from build123d import *

# Parameters (mm, degrees)
SKETCH1_W           = 40
SKETCH1_H           = 30
SKETCH1_W_2         = 34
SKETCH1_H_2         = 24
EXTRUDE_THIN1_DEPTH = 330
EXTRUDE1_DEPTH      = 41
EXTRUDE2_DEPTH      = 33.318373456


with BuildPart() as part:
    # Sketch1 → Extrude-Thin1 (new body)
    with BuildSketch(Plane(origin=(0, 0, 0), x_dir=(1, 0, 0), z_dir=(0, 1, 0))):
        Rectangle(SKETCH1_W, SKETCH1_H)
        Rectangle(SKETCH1_W_2, SKETCH1_H_2, mode=Mode.SUBTRACT)
    extrude(amount=EXTRUDE_THIN1_DEPTH)

    # Sketch2 → Extrude1 (cut, through all)
    with BuildSketch(Plane.ZY.offset(20)):
        Polygon((-15, 330), (15, 330), (15, 318.182685732), align=None)
    extrude(amount=-EXTRUDE1_DEPTH, mode=Mode.SUBTRACT)

    # Sketch3 → Extrude2 (cut, through all, along a direction that is not the sketch's normal)
    with BuildSketch(Plane(origin=(0, 0, -15), x_dir=(-1, 0, 0), z_dir=(0, 0, -1))):
        Polygon((20, 330), (-20, 330), (-20, 319.655296626), align=None)
    extrude(amount=-EXTRUDE2_DEPTH, dir=(0, 0.366501227, -0.930417568), mode=Mode.SUBTRACT)


solid = part.part
The listing builds one solid part. Answer for the finished solid, in the listing's coordinates (mm). A direction names the side the tool comes from. Coordinates: 2 decimals unless noted, no trailing zeros. Write each loop counter-clockwise with the first axis right and the second up, starting at its lowest first coordinate (ties: lowest second). Pieces come first, ordered by that corner, then holes. Notation, with made-up numbers: (-19, -20) - (24, -20) arc R19 ccw to (24, -7) - close; hole circle Ø6 at (41.5, 44). An arc over 180 degrees is marked (long way). Put each result on its own line as item: value.
1. The part is cut by section A-A on y = 181.5. Give the vertices of the cut face in (x, z), plus the area to 3 significant figures.
Answer sheet:
outline: (-20, -15) - (20, -15) - (20, 15) - (-20, 15) - close; hole (-17, -12) - (17, -12) - (17, 12) - (-17, 12) - close
area: 384 mm^2
2. Find the intervals of material crossed by line 1 along X through (y, z) = (164.5, -5.5); line 2 along Z through (x, y) = (15, 84); line 3 along Y through (x, z) = (17.5, 7.5), in increasing order. Write a range as from..to.
Answer sheet:
line 1: x = -20..-17, 17..20
line 2: z = -15..-12, 12..15
line 3: y = 0..311.44
3. The part is cut by section C-C on x = -3. Give the vertices of the cut face in (y, z), plus the area to 3 significant figures.
Answer sheet:
outline: (0, -15) - (325.6, -15) - (324.42, -12) - (0, -12) - close; (0, 12) - (314.97, 12) - (313.79, 15) - (0, 15) - close
area: 1,920 mm^2
4. A flat-ended cylindrical pin translates along its axis: pin 1 Ø8 at (x, z) = (-14, 0) entering from -Y. Find the tip coordinate at first contact, or state that the pin passes through.
Answer sheet:
pin 1: stops at y = 0
5. A tool of negligible diameter and unlimited length cuts with its end or side. For faces 4 (the face through (0, 162, -12)), 5 (the face through (-0.31, 323.84, -12.29)), from which of +Z, -Z, +X, -X, +Y, -Y can it reach the whole face along a straight path? Write none if from no direction.
Answer sheet:
face 4: +Y, -Y
face 5: +Z, +X, +Y
6. The part is cut by section B-B on z = 2.5. Give the vertices of the cut face in (x, y).
Answer sheet:
outline: (-20, 0) - (-17, 0) - (-17, 322.33) - (-20, 323.11) - close; (17, 0) - (20, 0) - (20, 312.76) - (17, 313.54) - close
7. Determine the mould class of faces 1 (the face through (20, 158, 0)), 2 (the face through (0, 157, 12)), 3 (the face through (0, 157, 15)) for opening direction Z: pulls with the +Z half, pulls with the -Z half, needs draft (parallel to the pull), parting line crosses it, or undercut.
Answer sheet:
face 1: needs draft
face 2: undercut
face 3: pulls with the +Z half
